Verification items for the finished model (mm, model axes). A direction names the side the tool comes from. Coordinates: 2 decimals unless noted, no trailing zeros. Write each loop counter-clockwise with the first axis right and the second up, starting at its lowest first coordinate (ties: lowest second). Pieces come first, ordered by that corner, then holes. Notation, with made-up numbers: (76, -17.75) -> (85, -17.75) arc R11 cw to (85, -9.75) -> close; hole circle Ø5 at (56, 9). An arc over 180 degrees is marked (long way). Use CSV: the item, a comma, the result in double quotes.
```python
from build123d import *

# Parameters (mm, degrees)
BOSS_EXTRUDE1_DEPTH = 12.7
FILLET1_R           = 6.35
FILLET2_R           = 1
CUT_EXTRUDE1_REACH  = 115.77
SKETCH2_R           = 2.2
CUT_EXTRUDE2_REACH  = 125.947
SKETCH3_R           = 2.2
FILLET3_R           = 0.5


with BuildPart() as part:
    # Sketch1 → Boss-Extrude1 (new body)
    # profile 1 of 3: a face of its own
    with BuildSketch(Plane.XY):
        Polygon((0, 0), (0, -101.6), (76.2, -101.6), align=None)
        Polygon((63.5, -95.25), (6.35, -19.05), (6.35, -95.25), align=None, mode=Mode.SUBTRACT)
    # profile 2 of 3: a face of its own
    with BuildSketch(Plane.XY):
        Polygon((34.925, -57.15), (6.35, -95.25), (8.85, -95.25), (36.175, -58.816666667), align=None)
    # profile 3 of 3: a face of its own
    with BuildSketch(Plane.XY):
        Polygon((33.675, -55.483333333), (6.35, -91.916666667), (6.35, -95.25), (34.925, -57.15), align=None)
    extrude(amount=BOSS_EXTRUDE1_DEPTH)

    # Fillet1
    fillet1_edges = [part.edges().sort_by_distance(p)[0] for p in [
        (0, 0, 6.35),
        (76.2, -101.6, 6.35),
        (0, -101.6, 6.35),
    ]]
    fillet(fillet1_edges, radius=FILLET1_R)

    # Fillet2
    fillet2_edges = [part.edges().sort_by_distance(p)[0] for p in [
        (36.175, -58.816666667, 6.35),
        (8.85, -95.25, 6.35),
        (63.5, -95.25, 6.35),
        (6.35, -19.05, 6.35),
        (6.35, -91.916666667, 6.35),
        (33.675, -55.483333333, 6.35),
    ]]
    fillet(fillet2_edges, radius=FILLET2_R)

    # Sketch2 → Cut-Extrude1 (cut, up to next)
    with BuildSketch(Plane.XZ.offset(101.6), mode=Mode.PRIVATE) as cut_extrude1_sk1:
        with Locations(Location((19.05, 6.35, 0), (0, 0, 270))):
            Circle(SKETCH2_R)
    cut_extrude1_tool1 = extrude(cut_extrude1_sk1.sketch, amount=-CUT_EXTRUDE1_REACH, mode=Mode.PRIVATE) & part.part
    # Sketch2 → Cut-Extrude1 (cut, up to next)
    with BuildSketch(Plane.XZ.offset(101.6), mode=Mode.PRIVATE) as cut_extrude1_sk2:
        with Locations(Location((44.45, 6.35, 0), (0, 0, 270))):
            Circle(SKETCH2_R)
    cut_extrude1_tool2 = extrude(cut_extrude1_sk2.sketch, amount=-CUT_EXTRUDE1_REACH, mode=Mode.PRIVATE) & part.part
    add(cut_extrude1_tool1.solids().sort_by_distance((19.05, -101.6, 6.35))[0], mode=Mode.SUBTRACT)
    add(cut_extrude1_tool2.solids().sort_by_distance((44.45, -101.6, 6.35))[0], mode=Mode.SUBTRACT)

    # Sketch3 → Cut-Extrude2 (cut, up to next)
    with BuildSketch(Plane.ZY, mode=Mode.PRIVATE) as cut_extrude2_sk1:
        with Locations(Location((6.35, -82.55, 0), (0, 0, 270))):
            Circle(SKETCH3_R)
    cut_extrude2_tool1 = extrude(cut_extrude2_sk1.sketch, amount=-CUT_EXTRUDE2_REACH, mode=Mode.PRIVATE) & part.part
    # Sketch3 → Cut-Extrude2 (cut, up to next)
    with BuildSketch(Plane.ZY, mode=Mode.PRIVATE) as cut_extrude2_sk2:
        with Locations(Location((6.35, -57.15, 0), (0, 0, 270))):
            Circle(SKETCH3_R)
    cut_extrude2_tool2 = extrude(cut_extrude2_sk2.sketch, amount=-CUT_EXTRUDE2_REACH, mode=Mode.PRIVATE) & part.part
    # Sketch3 → Cut-Extrude2 (cut, up to next)
    with BuildSketch(Plane.ZY, mode=Mode.PRIVATE) as cut_extrude2_sk3:
        with Locations(Location((6.35, -31.75, 0), (0, 0, 270))):
            Circle(SKETCH3_R)
    cut_extrude2_tool3 = extrude(cut_extrude2_sk3.sketch, amount=-CUT_EXTRUDE2_REACH, mode=Mode.PRIVATE) & part.part
    add(cut_extrude2_tool1.solids().sort_by_distance((0, -82.55, 6.35))[0], mode=Mode.SUBTRACT)
    add(cut_extrude2_tool2.solids().sort_by_distance((0, -57.15, 6.35))[0], mode=Mode.SUBTRACT)
    add(cut_extrude2_tool3.solids().sort_by_distance((0, -31.75, 6.35))[0], mode=Mode.SUBTRACT)

    # Fillet3
    fillet3_edges = [part.edges().sort_by_distance(p)[0] for p in [
        (34.925, -101.6, 0),
        (34.925, -101.6, 12.7),
        (0, -57.15, 0),
        (40.005, -53.34, 0),
        (69.179612663, -98.089806331, 0),
        (4.341953686, -13.025861057, 0),
        (1.859871939, -99.740128061, 0),
        (0, -57.15, 12.7),
        (40.005, -53.34, 12.7),
        (69.179612663, -98.089806331, 12.7),
        (4.341953686, -13.025861057, 12.7),
        (1.859871939, -99.740128061, 12.7),
    ]]
    fillet(fillet3_edges, radius=FILLET3_R)


solid = part.part
```
1) Mould release check, pull along X, two halves, no side actions. Record for faces 1 (the cylindrical face through (46.63, -98.47, 6.64)), 2 (the flat face through (25, -73, 12.7)), 3 (the flat face through (0, -57, 9)): released by +X, released by -X, zero draft, split by the parting line, or undercut.
Return value:
face 1,"undercut"
face 2,"zero draft"
face 3,"released by -X"
2) Gauge pin test, flat ends, axial feed: pin 1 (4 mm diameter, centred on x = 13, z = 5.5, fed in from +Y); pin 2 (6.5 mm diameter, centred on x = 38.5, z = 7.5, fed in from +Y); pin 3 (5 mm diameter, centred on y = -31.75, z = 6.35, fed in from +X). Record the tip position at first contact, or that the pin passes through.
Return value:
pin 1,"y = -14.73"
pin 2,"y = -47"
pin 3,"x = 25.69"
3) Cross-section at A-A (z = 10.5). Record the boundary of the cut face in (x, y) (3 decimals), plus the area to 3 significant figures.
Return value:
outline,"(0, -95.25) arc R6.35 ccw to (6.35, -101.6) -> (63.5, -101.6) arc R6.35 ccw to (68.58, -91.44) -> (11.43, -15.24) arc R6.35 ccw to (0, -19.05) -> close; hole (6.35, -88.917) arc R1 ccw to (8.15, -89.517) -> (33.225, -56.083) arc R1 ccw to (33.225, -54.883) -> (8.15, -21.45) arc R1 ccw to (6.35, -22.05) -> close; hole (10.05, -93.65) arc R1 ccw to (10.85, -95.25) -> (61.5, -95.25) arc R1 ccw to (62.3, -93.65) -> (36.975, -59.883) arc R1 ccw to (35.375, -59.883) -> close"
area,"1,770 mm2"
4) Cross-section at B-B (z = 6.35). Give the number of separate pieces and of enclosed holes in the cut face, plus the area to 3 significant figures.
Return value:
separate pieces,"4"
enclosed holes,"0"
area,"1,630 mm2"
5) Set-up check for faces 4 (the flat face through (49.81, -77, 6.26)), 5 (the cylindrical face through (3.131, -55.404, 5.011)), 6 (the cylindrical face through (17.1, -98.47, 5.33)): record each of +Z, -Z, +X, -X, +Y, -Y from which the full face is reachable in a straight line by a thin tool's end or side.
Return value:
face 4,"+Z, -Z"
face 5,"-X"
face 6,"-Y"
6) Scan lines: L1, parallel to Z at x = 2, y = -57; L2, parallel to X at y = -99, z = 6.35; L3, parallel to X at y = -100, z = 6.35. Record each from-to range of solid material in increasing order.
Return value:
L1,"0 to 4.16, 8.54 to 12.7"
L2,"1.23 to 16.85, 21.25 to 42.25, 46.65 to 68.62"
L3,"2.14 to 16.85, 21.25 to 42.25, 46.65 to 67.71"
